Verification items for the finished model (mm, model axes). A direction names the side the tool comes from. Round coordinates to 2 decimals unless told otherwise and drop trailing zeros. Loops run counter-clockwise (first coordinate to the right, second up) from the corner with the lowest first, then second, coordinate; pieces in that order, holes last. Notation, with made-up numbers: (66, 69) -> (95, 69) arc R28 ccw to (95, 105) -> close; hole circle Ø7 at (-32, 41). An arc over 180 degrees is marked (long way). Write item = value, one per line. Start each with the question number.
```python
from build123d import *

# Parameters (mm, degrees)
EXTRUDE_1_DEPTH     = 3
SKETCH_2_W          = 18
SKETCH_2_H          = 14
SKETCH_2_H_2        = 16
SKETCH_2_W_2        = 15
CUT_EXTRUDE_1_DEPTH = 10
FILLET_1_R          = 2
FILLET_2_R          = 3
SKETCH_4_R          = 2.025
CUT_EXTRUDE_2_DEPTH = 10
SKETCH_5_R          = 2.025
CUT_EXTRUDE_3_DEPTH = 10


with BuildPart() as part:
    # 草图1 → 凸台-拉伸1 (new body)
    with BuildSketch(Plane.XY):
        Polygon((0, 0), (60, 0), (60, -30), (30, -60), (0, -60), align=None)
    extrude(amount=EXTRUDE_1_DEPTH)

    # 草图2 → 切除-拉伸1 (cut)
    with BuildSketch(Plane.XY.offset(3)):
        Polygon((30, -51.514718626), (30, -30), (51.514718626, -30), align=None)
        with Locations((15, -15)):
            Rectangle(SKETCH_2_W, SKETCH_2_H)
        with Locations((15, -44)):
            Rectangle(SKETCH_2_W, SKETCH_2_H_2)
        with Locations((45.5, -15)):
            Rectangle(SKETCH_2_W_2, SKETCH_2_H)
    extrude(amount=-CUT_EXTRUDE_1_DEPTH, mode=Mode.SUBTRACT)

    # 圆角1
    fillet_1_edges = [part.edges().sort_by_distance(p)[0] for p in [
        (53, -8, 1.5),
        (53, -22, 1.5),
        (38, -22, 1.5),
        (38, -8, 1.5),
        (51.514718626, -30, 1.5),
        (30, -51.514718626, 1.5),
        (30, -30, 1.5),
        (24, -36, 1.5),
        (24, -52, 1.5),
        (6, -52, 1.5),
        (6, -36, 1.5),
        (24, -8, 1.5),
        (24, -22, 1.5),
        (6, -22, 1.5),
        (6, -8, 1.5),
    ]]
    fillet(fillet_1_edges, radius=FILLET_1_R)

    # 圆角2
    fillet_2_edges = [part.edges().sort_by_distance(p)[0] for p in [
        (0, 0, 1.5),
        (60, 0, 1.5),
        (60, -30, 1.5),
        (30, -60, 1.5),
        (0, -60, 1.5),
    ]]
    fillet(fillet_2_edges, radius=FILLET_2_R)

    # 草图4 → 切除-拉伸2 (cut)
    with BuildSketch(Plane.XY.offset(3)):
        with Locations((15, -29)):
            Circle(SKETCH_4_R)
        with Locations((15, -56)):
            Circle(SKETCH_4_R)
        with Locations((15, -4)):
            Circle(SKETCH_4_R)
    extrude(amount=-CUT_EXTRUDE_2_DEPTH, mode=Mode.SUBTRACT)

    # 草图5 → 切除-拉伸3 (cut)
    with BuildSketch(Plane.XY.offset(3)):
        with Locations((34, -15)):
            Circle(SKETCH_5_R)
        with Locations((56.5, -15)):
            Circle(SKETCH_5_R)
    extrude(amount=-CUT_EXTRUDE_3_DEPTH, mode=Mode.SUBTRACT)


solid = part.part
```
(1) Draft check along X on faces 1 (the cylindrical face through (23.43, -51.4, 1.48)), 2 (the flat face through (0, -30, 1)), 3 (the flat face through (38, -15, 2)), 4 (the flat face through (30, 0, 1)). Enter one of: +X half, -X half, draft (parallel to the pull), parting line (faces both ways), or undercut.
(2) Section check A-A on y = -56. Enter the section's corners in (x, z) (3 decimals), then the cut area to 4 significant figures.
(3) Scan lines: line 1 (Y direction, x = 18, z = 1.35); line 2 (X direction, y = -10, z = 1.9); line 3 (Y direction, x = 6.5, z = 1.5). Record each from-to range of solid material in increasing order. Write a range as [from, to].
(4) Access from +Z, -Z, +X, -X, +Y, -Y to the whole of each face (thin tool, end or side, straight path). Record for faces 5 (the flat face through (30, -23, 0)), 6 (the cylindrical face through (48.52, -31.2, 1.48)).
(5) Section check B-B on x = 10.5. Enter the section's corners in (y, z), then the cut area to 3 significant figures.
(6) Depth check by flat-ended pin: pin 1 Ø0.9 at (x, z) = (38, 2) entering from -Y. Enter the tip coordinate at first touch or a pass-through.
(7) Section check C-C on y = -15. Enter the section's corners in (x, z) (3 decimals).
(8) Section check D-D on y = -41.5. Enter the section's corners in (x, z).
Computed values:
q1.face_1 = undercut
q1.face_2 = -X half
q1.face_3 = undercut
q1.face_4 = draft
q2.outline = (0, 0) -> (12.975, 0) -> (12.975, 3) -> (0, 3) -> close; (17.025, 0) -> (34, 0) -> (34, 3) -> (17.025, 3) -> close
q2.area = 89.85 mm²
q3.line_1 = [-60, -52], [-36, -22], [-8, 0]
q3.line_2 = [0, 6], [24, 38], [53, 60]
q3.line_3 = [-60, -51.32], [-36.68, -21.32], [-8.68, 0]
q4.face_5 = -Z, +X, -X, +Y, -Y
q4.face_6 = +Z, -Z
q5.outline = (-60, 0) -> (-52, 0) -> (-52, 3) -> (-60, 3) -> close; (-36, 0) -> (-22, 0) -> (-22, 3) -> (-36, 3) -> close; (-8, 0) -> (0, 0) -> (0, 3) -> (-8, 3) -> close
q5.area = 90.0 mm²
q6.pin_1 = -52.45
q7.outline = (0, 0) -> (6, 0) -> (6, 3) -> (0, 3) -> close; (24, 0) -> (31.975, 0) -> (31.975, 3) -> (24, 3) -> close; (36.025, 0) -> (38, 0) -> (38, 3) -> (36.025, 3) -> close; (53, 0) -> (54.475, 0) -> (54.475, 3) -> (53, 3) -> close; (58.525, 0) -> (60, 0) -> (60, 3) -> (58.525, 3) -> close
q8.outline = (0, 0) -> (6, 0) -> (6, 3) -> (0, 3) -> close; (24, 0) -> (30, 0) -> (30, 3) -> (24, 3) -> close; (40.01, 0) -> (48.5, 0) -> (48.5, 3) -> (40.01, 3) -> close
